from build123d import *

# Parameters (mm, degrees)
F2_R     = 10
F3_DEPTH = 27.4852500417
F4_R     = 1.8315852812
F4_R_2   = 2.4433835159
F5_DEPTH = 27.5293034423


with BuildPart() as f1:
    # F0 (on Front) → F1 (revolve)
    with BuildSketch(Plane.XZ):
        with BuildLine():
            Line((-27.533114626, 0), (27.533114626, 0))
            ThreePointArc((27.533114626, 0), (0, 27.533114626), (-27.533114626, 0))
        make_face()
    revolve(axis=Axis((6.374521181, 0, 0), (1, 0, 0)))

    # F2 (on Front) → F3 (cut, through all)
    with BuildSketch(Plane.XZ):
        Circle(F2_R)
        with BuildLine():
            ThreePointArc((-1.5828419389, 0.4278055021), (0, 6.193420209), (1.5828419389, 0.4278055021))
            ThreePointArc((1.5828419389, 0.4278055021), (0, -6.6799922122), (-1.5828419389, 0.4278055021))
        make_face(mode=Mode.SUBTRACT)
    extrude(amount=F3_DEPTH, mode=Mode.SUBTRACT)

    # F4 (on Front) → F5 (cut, through all)
    with BuildSketch(Plane.XZ):
        with Locations((0, 3.1033086125)):
            Circle(F4_R)
        with Locations((0, -2.9580835253)):
            Circle(F4_R_2)
    extrude(amount=F5_DEPTH, mode=Mode.SUBTRACT)


solid = f1.part
Read the model definition and answer for the solid it produces. Units are mm, in the model's axes. Give positions to 0.01 mm unless a question says otherwise; leave off trailing zeros. Write each loop counter-clockwise with the first axis right and the second up, starting at its lowest first coordinate (ties: lowest second). Pieces come first, ordered by that corner, then holes. Notation, with made-up numbers: (79, 17.25) - (124, 17.25) arc R28 ccw to (124, 52.25) - close; hole circle Ø10 at (55, 68.25). An arc over 180 degrees is marked (long way). Use CSV: the item, a comma, the result in double quotes. Start each with the question number.
(1) Determine the mould class of faces 1 (the cylindrical face through (-0.397, -13.559, 1.315)), 2 (the cylindrical face through (0.141, -13.55, -6.677)) for opening direction X: +X half, -X half, draft (parallel to the pull), parting line (faces both ways), or undercut.
(2) Find section D-D (x = -7.5). Give the vertices of the cut face in (y, z), plus the area to 3 significant figures.
(3) Find section C-C (x = -20). Give the vertices of the cut face in (y, z), plus the area to 3 significant figures.
(4) Find section A-A (x = 0). Give the vertices of the cut face in (y, z), plus the area to 3 significant figures.
(5) Consider line 1 along Z through (x, y) = (0, -6.5); line 2 along Z through (x, y) = (0, -17.25); line 3 along Z through (x, y) = (8, -20). Determine where each line is inside the solid, lowest interval first.
(6) Find section B-B (y = 18). Give the vertices of the cut face in (x, z).
(7) Given P1, Ø12, axis at x = -14, y = 10, coming from the +Z side; P2, Ø5.5, axis at x = 0, z = -2.96, coming from the +Y side; P3, Ø1, axis at x = -13.5, z = -4, coming from the -Y side, each flat-ended and moving along its own axis, determine where each tip first touches the part or whether it passes through.
Findings below:
1,face 1,"undercut"
1,face 2,"undercut"
2,outline,"(-25.65, -6.61) arc R26.49 ccw (long way) to (-25.65, 6.61) - (0, 6.61) - (0, -6.61) - close"
2,area,"1,860 mm2"
3,outline,"circle Ø37.85 at (0, 0)"
3,area,"1,120 mm2"
4,outline,"(-27.53, -0.51) - (0, -0.51) - (0, -5.4) - (-27, -5.4) arc R27.53 ccw to (-26.71, -6.68) - (0, -6.68) - (0, -10) - (-25.65, -10) arc R27.53 ccw (long way) to (-25.65, 10) - (0, 10) - (0, 6.19) - (-26.83, 6.19) arc R27.53 ccw to (-27.09, 4.93) - (0, 4.93) - (0, 1.27) - (-27.5, 1.27) arc R27.53 ccw to start"
4,area,"1,960 mm2"
5,line 1,"-26.75 to -10, -6.68 to -5.4, -0.51 to 1.27, 4.93 to 6.19, 10 to 26.75"
5,line 2,"-21.46 to -10, -6.68 to -5.4, -0.51 to 1.27, 4.93 to 6.19, 10 to 21.46"
5,line 3,"-17.15 to -6, 6 to 17.15"
6,outline,"circle Ø41.67 at (0, 0)"
7,P1,"z = 25.15"
7,P2,"y = 27.53"
7,P3,"y = -23.95"
